Source: three-view drawing plus pictorial views. Frame: mm from the lowest corner of the part. Round coordinates to 2 decimals unless told otherwise and drop trailing zeros. Loops run counter-clockwise (first coordinate to the right, second up) from the corner with the lowest first, then second, coordinate; pieces in that order, holes last. Notation, with made-up numbers: (-11.5, 48) -> (40.5, 48) arc R33 cw to (40.5, 87) -> close; hole circle Ø11 at (-1, 3). An arc over 180 degrees is marked (long way). One line per question, with ' | ' between items. Start each with the question number.
Q1. Cut plane D-D on x = 50.8. Return loops of the section in (y, z).
Q2. Cut plane C-C on y = 2.1. Return loops of the section in (x, z) (1 decimal), and give its area (3 significant figures).
Q3. Contact query for flat-ended pins moving along their axis: P1, Ø6, axis at x = 90, z = 7.5, coming from the -Y side; P2, Ø1.3, axis at x = 73.5, y = 1, coming from the -Z side. Output: stop coordinate, or through.
Q4. Cut plane B-B on z = 11.5. Return loops of the section in (x, y).
Q5. Material intervals for L1, parallel to X at y = 0.4, z = 6.5; L2, parallel to X at y = 0.6, z = 25.5 (1 decimal); L3, parallel to X at y = 2.25, z = 22.5, sorted ascending.
Q6. Cut plane A-A on x = 97.17. Return loops of the section in (y, z).
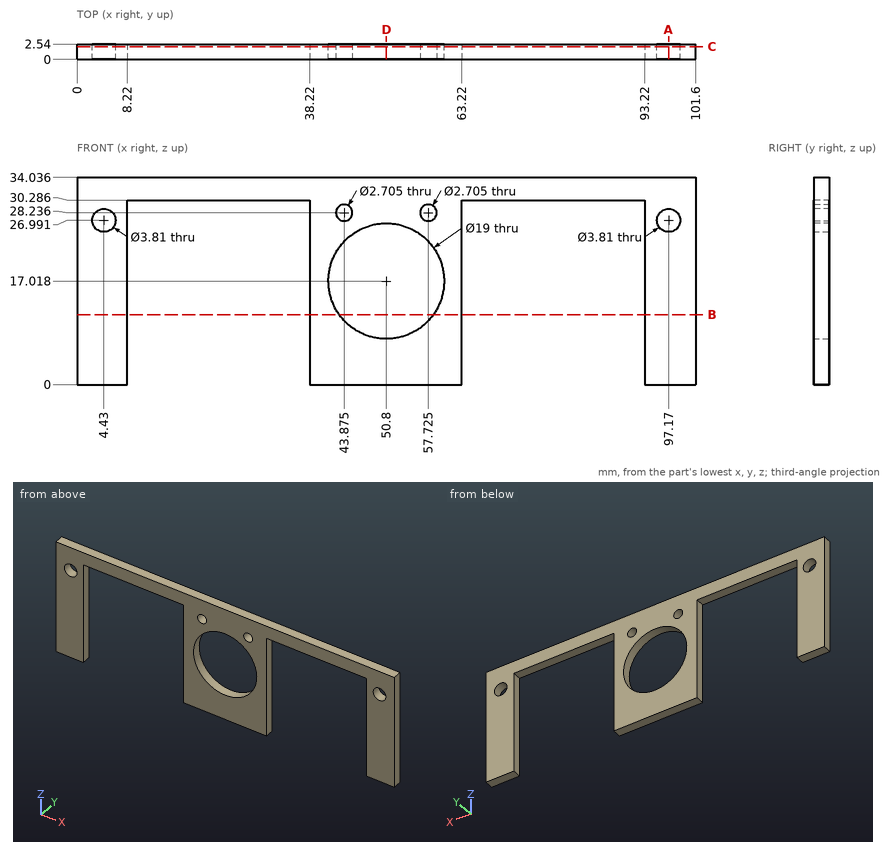
Results:
1) outline: (0, 0) -> (2.54, 0) -> (2.54, 7.52) -> (0, 7.52) -> close; (0, 26.52) -> (2.54, 26.52) -> (2.54, 34.04) -> (0, 34.04) -> close
2) outline: (0, 0) -> (8.2, 0) -> (8.2, 30.3) -> (38.2, 30.3) -> (38.2, 0) -> (63.2, 0) -> (63.2, 30.3) -> (93.2, 30.3) -> (93.2, 0) -> (101.6, 0) -> (101.6, 34) -> (0, 34) -> close; hole circle Ø3.8 at (4.4, 27); hole circle Ø19 at (50.8, 17); hole circle Ø2.7 at (43.9, 28.2); hole circle Ø2.7 at (57.7, 28.2); hole circle Ø3.8 at (97.2, 27) | area: 1,320 mm^2
3) P1: through | P2: z = 30.29
4) outline: (0, 0) -> (8.22, 0) -> (8.22, 2.54) -> (0, 2.54) -> close; (38.22, 0) -> (43.07, 0) -> (43.07, 2.54) -> (38.22, 2.54) -> close; (58.53, 0) -> (63.22, 0) -> (63.22, 2.54) -> (58.53, 2.54) -> close; (93.22, 0) -> (101.6, 0) -> (101.6, 2.54) -> (93.22, 2.54) -> close
5) L1: 0 to 8.22, 38.22 to 63.22, 93.22 to 101.6 | L2: 0 to 3.2, 5.6 to 8.2, 38.2 to 46.5, 55.1 to 63.2, 93.2 to 96, 98.4 to 101.6 | L3: 0 to 8.22, 38.22 to 43.04, 58.56 to 63.22, 93.22 to 101.6
6) outline: (0, 0) -> (2.54, 0) -> (2.54, 25.09) -> (0, 25.09) -> close; (0, 28.9) -> (2.54, 28.9) -> (2.54, 34.04) -> (0, 34.04) -> close
